```python
from build123d import *

# Parameters (mm, degrees)
SKETCH_3_R          = 1.25
CUT_EXTRUDE_1_DEPTH = 18.300578025
CHAMFER_1_SIZE      = 0.4


with BuildPart() as part:
    # Эскиз2 → Повернуть1 (revolve)
    with BuildSketch(Plane.XY, mode=Mode.PRIVATE) as revolve_1_sk:
        Polygon((0, 0), (0, 9.5), (-3.6, 9.5), (-3.6, 3.5), (-14.5, 3.5), (-14.5, 0), align=None)
    revolve(revolve_1_sk.sketch.rotate(Axis((-14.5, 0, 0), (1, 0, 0)), 90), axis=Axis((-14.5, 0, 0), (1, 0, 0)))

    # Эскиз3 → Вырез-Вытянуть1 (cut, through all)
    with BuildSketch(Plane.ZY.offset(3.6)):
        with Locations((0, 4.8)):
            Circle(SKETCH_3_R)
    extrude(amount=-CUT_EXTRUDE_1_DEPTH, mode=Mode.SUBTRACT)

    # Фаска1
    chamfer_1_edges = [part.edges().sort_by_distance(p)[0] for p in [
        (-14.5, 0, -3.5),
        (-3.6, 0, -9.5),
        (0, 0, -9.5),
    ]]
    chamfer(chamfer_1_edges, length=CHAMFER_1_SIZE)


solid = part.part
```
Geometry: final body of the model. Coordinates: model frame, mm. A direction names the side the tool comes from. Coordinates: 2 decimals unless noted, no trailing zeros. Loops run counter-clockwise (first coordinate to the right, second up) from the corner with the lowest first, then second, coordinate; pieces in that order, holes last. Notation, with made-up numbers: (74.5, 36) -> (105.5, 36) arc R15 ccw to (105.5, 44) -> close; hole circle Ø3 at (75, 15). An arc over 180 degrees is marked (long way). Use a Markdown table: item, result. Add a question column.
(1) Line query: line 1 along Y through (x, z) = (-1.5, 0); line 2 along X through (y, z) = (-4.5, -5.75); line 3 along Y through (x, z) = (-5.5, -1). Output: solid intervals per line, ascending.
(2) Pin query (flat end, axial travel): pin 1 Ø4 at (x, z) = (-7.5, -4) entering from +Y; pin 2 Ø2 at (y, z) = (4.8, 0) entering from -X; pin 3 Ø5 at (x, y) = (-8, 2.5) entering from +Z; pin 4 Ø2 at (x, z) = (-12.5, -2.5) entering from +Y. Return the tip coordinate at first contact, or that it passes through.
(3) Section query A-A, the plane z = 0. Return loops of the section in (x, y), plus the area to 3 significant figures.
(4) Section query C-C, the plane x = -1. Return loops of the section in (y, z), plus the area to 3 significant figures.
(5) Section query B-B, the plane y = 0. Return loops of the section in (x, z).
(6) Section query D-D, the plane x = -9.75. Return loops of the section in (y, z).
(7) Access query for faces 1 (the cylindrical face through (-1.83, 6.04, -0.16)), 2 (the cylindrical face through (-8.924, 3.105, 1.615)). Directions: +Z, -Z, +X, -X, +Y, -Y. A direction counts if a zero-diameter tool reaches every point of the face in a straight line with its end or side. Return the directions, or none.
Answer:
| question | item | result |
|---|---|---|
| 1 | line 1 | y = -9.5 to 3.55, 6.05 to 9.5 |
| 1 | line 2 | x = -3.6 to 0 |
| 1 | line 3 | y = -3.35 to 3.35 |
| 2 | pin 1 | stops at y = 2.87 |
| 2 | pin 2 | passes through |
| 2 | pin 3 | stops at z = 3.5 |
| 2 | pin 4 | stops at y = 3.16 |
| 3 | outline | (-14.5, -3.1) -> (-14.1, -3.5) -> (-3.6, -3.5) -> (-3.6, -9.1) -> (-3.2, -9.5) -> (-0.4, -9.5) -> (0, -9.1) -> (0, 3.55) -> (-3.6, 3.55) -> (-3.6, 3.5) -> (-14.1, 3.5) -> (-14.5, 3.1) -> close; (-3.6, 6.05) -> (0, 6.05) -> (0, 9.1) -> (-0.4, 9.5) -> (-3.2, 9.5) -> (-3.6, 9.1) -> close |
| 3 | area | 135 mm^2 |
| 4 | outline | circle Ø19 at (0, 0); hole circle Ø2.5 at (4.8, 0) |
| 4 | area | 279 mm^2 |
| 5 | outline | (-14.5, -3.1) -> (-14.1, -3.5) -> (-3.6, -3.5) -> (-3.6, -9.1) -> (-3.2, -9.5) -> (-0.4, -9.5) -> (0, -9.1) -> (0, 9.1) -> (-0.4, 9.5) -> (-3.2, 9.5) -> (-3.6, 9.1) -> (-3.6, 3.5) -> (-14.1, 3.5) -> (-14.5, 3.1) -> close |
| 6 | outline | circle Ø7 at (0, 0) |
| 7 | face 1 | +X, -X |
| 7 | face 2 | -X |
